Work out the finished part from the listing and answer in its coordinate system (mm). A direction names the side the tool comes from. Give positions to 0.01 mm unless a question says otherwise; leave off trailing zeros. Write each loop counter-clockwise with the first axis right and the second up, starting at its lowest first coordinate (ties: lowest second). Pieces come first, ordered by that corner, then holes.
1) Given pin 1 Ø3 at (x, z) = (8.5, 6) entering from -Y; pin 2 Ø1.2 at (y, z) = (27, 5) entering from -X; pin 3 Ø4 at (y, z) = (9, 4) entering from +X; pin 4 Ø1.5 at (x, z) = (6.5, 4) entering from +Y, each flat-ended and moving along its own axis, determine where each tip first touches the part or whether it passes through.
2) Determine the mould class of faces 1 (the face through (-1, 7, 10)), 2 (the face through (-0.986, 26.263, 5.676)), 3 (the face through (-1, 32, 5)) for opening direction Z: pulls with the +Z half, pulls with the -Z half, needs draft (parallel to the pull), parting line crosses it, or undercut.
3) Straight lines are drawn through the part: probe 1 along Z at (x, y) = (-1.2, 27); probe 2 along X at (y, z) = (10, 3); probe 3 along X at (y, z) = (-7, 4.5). For each, find the intervals that lie inside material, in ascending order.
4) Find section D-D (y = -5). Determine the outline of the cut face in (x, z), plus the area to 3 significant figures.
5) Find section B-B (y = 27). Determine the outline of the cut face in (x, z).
6) Find section A-A (z = 5). Determine the outline of the cut face in (x, y).
7) A tool of negligible diameter and unlimited length cuts with its end or side. For faces 4 (the face through (-1, 4, 5)), 5 (the face through (-2, 14.8, 3.8)), 6 (the face through (0, 17, 5)), 7 (the face through (19, -14, 5)), 8 (the face through (7, -2, 5)), from which of +Z, -Z, +X, -X, +Y, -Y can it reach the whole face along a straight path? Write none if from no direction.
8) Find section C-C (x = 13.5). Determine the outline of the cut face in (y, z).
Autodesk Fusion 360 part; units mm, degrees
sketch "Sketch2" plane through (0, 0, 0) normal (0, 0, 1) x (1, 0, 0)
  line L0 (0, 0) -> (-2, 0)
  line L1 (-2, 0) -> (-2, 32)
  line L2 (-2, 32) -> (0, 32)
  line L3 (0, 32) -> (0, 0)
  line L4 (-2, 0) -> (18, 0)
  line L5 (18, 0) -> (18, -2)
  line L6 (18, -2) -> (-2, -2)
  line L7 (-2, -2) -> (-2, 0)
  line L8 (18, 0) -> (20, 0)
  line L9 (20, 0) -> (20, -14)
  line L10 (20, -14) -> (18, -14)
  line L11 (18, -14) -> (18, 0)
  dimension "d5" = 2
  dimension "d6" = 32
  dimension "d7" = 20
  dimension "d8" = 2
  dimension "d9" = 2
  dimension "d10" = 14
extrude "Extrude1" add sketch "Sketch2" along normal blind 10
sketch "Sketch3" plane through (0, 0, 0) normal (1, 0, 0) x (0, 1, 0)
  line L0 (0, 0) -> (32, 0)
  line L1 (32, 0) -> (32, 10)
  line L2 (32, 10) -> (0, 10)
  line L3 (0, 10) -> (0, 0)
  circle A0 centre (27, 5) radius 1
  circle A1 centre (15, 5) radius 1
  circle A2 centre (5, 5) radius 1
  line L4 (5, 6) -> (15, 6)
  line L5 (15, 6) -> (15, 4)
  line L6 (15, 4) -> (5, 4)
  line L7 (5, 4) -> (5, 6)
  dimension "d15" = 2
  dimension "d16" = 5
  dimension "d17" = 5
  dimension "d18" = 2
  dimension "d19" = 15
  dimension "d20" = 2
  dimension "d21" = 5
  dimension "d22" = 5
  dimension "d23" = 5
  dimension "d24" = 2
extrude "Extrude2" cut sketch "Sketch3" against normal blind 2 contours A0 | A1 L5 | A1 L5 | A1 A2 L4 L6 | A2 L7 | A2 L7
fillet "Fillet1" radius 2 1 edges at (0, 0, 5)
fillet "Fillet1" radius 2 1 edges at (18, -2, 5)
fillet "Fillet1" radius 1 1 edges at (20, 0, 5)
equation "thickness = 2 mm"
equation "d5 = thickness"
equation "d7 = window_depth"
equation "d8 = thickness"
equation "d9 = thickness"
equation "width = 10 mm"
equation "d12 = width"
equation "hole = 2 mm"
equation "d15 = hole"
equation "d16 = width / 2"
equation "d17 = width / 2"
equation "d18 = hole"
equation "d19 = width + width / 2"
equation "d20 = hole"
equation "d21 = width / 2"
equation "d22 = width / 2"
equation "d23 = width / 2"
equation "d24 = hole"
equation "d28 = thickness"
equation "d30 = thickness"
equation "d32 = thickness / 2"
equation "window_depth = 20 mm"
Results:
1. pin 1: stops at y = -2
1. pin 2: passes through
1. pin 3: stops at x = 0
1. pin 4: stops at y = 0
2. face 1: pulls with the +Z half
2. face 2: undercut
2. face 3: needs draft
3. probe 1: z = 0 to 4, 6 to 10
3. probe 2: x = -2 to 0
3. probe 3: x = 18 to 20
4. outline: (18, 0) - (20, 0) - (20, 10) - (18, 10) - close
4. area: 20.0 mm2
5. outline: (-2, 0) - (0, 0) - (0, 4) - (-2, 4) - close; (-2, 6) - (0, 6) - (0, 10) - (-2, 10) - close
6. outline: (-2, -2) - (16, -2) arc R2 cw to (18, -4) - (18, -14) - (20, -14) - (20, -1) arc R1 ccw to (19, 0) - (2, 0) arc R2 cw to (0, 2) - (0, 4) - (-2, 4) - close; (-2, 16) - (0, 16) - (0, 26) - (-2, 26) - close; (-2, 28) - (0, 28) - (0, 32) - (-2, 32) - close
7. face 4: +X, -X
7. face 5: +Z, -Z, -X, +Y, -Y
7. face 6: +Z, -Z, +X, +Y
7. face 7: +Z, -Z, +X, -X, -Y
7. face 8: +Z, -Z, -X, -Y
8. outline: (-2, 0) - (0, 0) - (0, 10) - (-2, 10) - close
